Can you work these out from the model? Positions are in its coordinate system, mm. Face numbers are marked on the shaded views. A direction names the side the tool comes from. Round coordinates to 2 decimals unless told otherwise and drop trailing zeros. Write each loop counter-clockwise with the first axis right and the second up, starting at its lowest first coordinate (ties: lowest second). Pieces come first, ordered by that corner, then holes.
Q1. If we section it at A-A (y = 0): Please give me the cut outline in (x, z).
Q2. For the marked faces 1, 2, 3, 4 and 5, which set-ups out of +Z, -Z, +X, -X, +Y, -Y let a thin tool reach every point of the face, with its end or its side?
Q3. We'd pull the mould along Y, two halves only. Please class the marked faces 6, 7 and 8: +Y half, -Y half, draft (parallel to the pull), parting line (faces both ways), or undercut.
Q4. I'm going to push flat-ended pins straight in: pin 1 Ø5 at (x, z) = (0.5, 7) entering from -Y; pin 2 Ø7 at (y, z) = (3.5, 10) entering from -X; pin 3 Ø8 at (x, y) = (16.5, 15.5) entering from +Z; pin 4 Ø4 at (y, z) = (1.5, 5) entering from -X. Where does each tip first touch, or does it pass through?
Q5. If we section it at B-B (z = 10.75): Please give me the cut outline in (x, y), plus the area to 3 significant figures.
Q6. If we section it at D-D (z = 3): Please give me the cut outline in (x, y), plus the area to 3 significant figures.
Q7. Please list where these lines run through material, in increasing order: line 1 along X through (y, z) = (-2.5, 10.25); line 2 along Z through (x, y) = (8.5, 15).
from build123d import *

# Parameters (mm, degrees)
BOX001_W        = 10.2
BOX001_H        = 10.2
BOX001_DEPTH    = 12.5
CHAMFER002_SIZE = 2
BOX_W           = 20
BOX_H           = 20
BOX_DEPTH       = 10
CHAMFER_SIZE    = 6
CHAMFER001_SIZE = 2
FILLET001_R     = 1
CYLINDER_R      = 25
CYLINDER_DEPTH  = 5
FILLET_R        = 1
FILLET002_R     = 1


with BuildPart() as chamfered_hole:
    # Box001 → Box001 (new body)
    with BuildSketch(Plane(origin=(-5.1, -5.1, 0), x_dir=(1, 0, 0), z_dir=(0, 0, 1))):
        with Locations((5.1, 5.1)):
            Rectangle(BOX001_W, BOX001_H)
    extrude(amount=BOX001_DEPTH)

    # Chamfer002
    chamfer002_edges = [chamfered_hole.edges().sort_by_distance(p)[0] for p in [
        (-5.1, -5.1, 6.25),
        (-5.1, 5.1, 6.25),
        (5.1, -5.1, 6.25),
        (5.1, 5.1, 6.25),
    ]]
    chamfer(chamfer002_edges, length=CHAMFER002_SIZE)


with BuildPart() as fillet001:
    # Box → Box (new body)
    with BuildSketch(Plane(origin=(-10, -10, 5), x_dir=(1, 0, 0), z_dir=(0, 0, 1))):
        with Locations((10, 10)):
            Rectangle(BOX_W, BOX_H)
    extrude(amount=BOX_DEPTH)

    # Chamfer
    chamfer_edges = [fillet001.edges().sort_by_distance(p)[0] for p in [
        (-10, -10, 10),
        (10, -10, 10),
    ]]
    chamfer(chamfer_edges, length=CHAMFER_SIZE)

    # Chamfer001
    chamfer001_edges = [fillet001.edges().sort_by_distance(p)[0] for p in [
        (-10, 10, 10),
        (10, 10, 10),
    ]]
    chamfer(chamfer001_edges, length=CHAMFER001_SIZE)

    # Fillet001
    fillet001_edges = [fillet001.edges().sort_by_distance(p)[0] for p in [
        (-10, 2, 15),
        (-9, 9, 15),
        (-7, -7, 15),
        (0, 10, 15),
        (0, -10, 15),
        (9, 9, 15),
        (7, -7, 15),
        (10, 2, 15),
    ]]
    fillet(fillet001_edges, radius=FILLET001_R)


with BuildPart() as print2_side_with_support:
    # Cylinder → Cylinder (new body)
    with BuildSketch(Plane.XY):
        Circle(CYLINDER_R)
    extrude(amount=CYLINDER_DEPTH)

    # Fillet
    fillet_edges = [print2_side_with_support.edges().sort_by_distance(p)[0] for p in [
        (-25, 0, 5),
        (-25, 0, 0),
    ]]
    fillet(fillet_edges, radius=FILLET_R)

    # Fusion: union Fillet001
    add(fillet001.part)

    # Cut: cut Chamfered hole
    add(chamfered_hole.part, mode=Mode.SUBTRACT)

    # Fillet002
    fillet002_edges = [print2_side_with_support.edges().sort_by_distance(p)[0] for p in [
        (0, -5.1, 0),
        (4.1, -4.1, 0),
        (5.1, 0, 0),
        (4.1, 4.1, 0),
        (0, 5.1, 0),
        (-4.1, 4.1, 0),
        (-5.1, 0, 0),
        (-4.1, -4.1, 0),
    ]]
    fillet(fillet002_edges, radius=FILLET002_R)


solid = print2_side_with_support.part
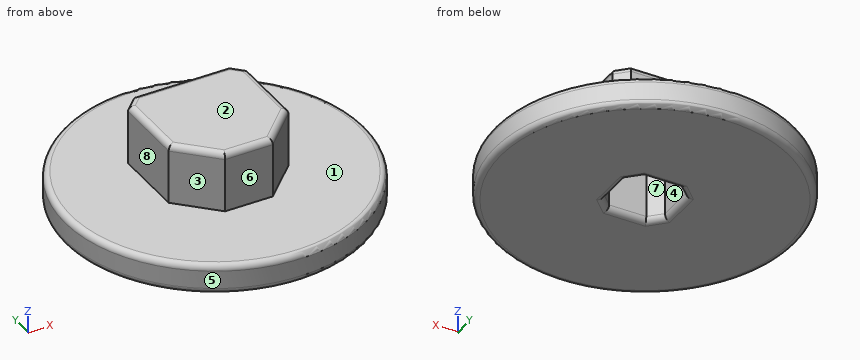
A:
1. outline: (-25, 1) arc R1 ccw to (-24, 0) - (-6.1, 0) arc R1 ccw to (-5.1, 1) - (-5.1, 12.5) - (5.1, 12.5) - (5.1, 1) arc R1 ccw to (6.1, 0) - (24, 0) arc R1 ccw to (25, 1) - (25, 4) arc R1 ccw to (24, 5) - (10, 5) - (10, 14) arc R1 ccw to (9, 15) - (-9, 15) arc R1 ccw to (-10, 14) - (-10, 5) - (-24, 5) arc R1 ccw to (-25, 4) - close
2. face 1: +Z
2. face 2: +Z, +X, -X, +Y, -Y
2. face 3: +Z, -X, -Y
2. face 4: -Z
2. face 5: +Z, -Z
3. face 6: -Y half
3. face 7: undercut
3. face 8: draft
4. pin 1: stops at y = -24.86
4. pin 2: stops at x = -10
4. pin 3: stops at z = 5
4. pin 4: stops at x = -25
5. outline: (-10, -4) - (-4, -10) - (4, -10) - (10, -4) - (10, 8) - (8, 10) - (-8, 10) - (-10, 8) - close; hole (-5.1, -3.1) - (-3.1, -5.1) - (3.1, -5.1) - (5.1, -3.1) - (5.1, 3.1) - (3.1, 5.1) - (-3.1, 5.1) - (-5.1, 3.1) - close
5. area: 264 mm2
6. outline: circle Ø50 at (0, 0); hole (-5.1, -3.1) - (-3.1, -5.1) - (3.1, -5.1) - (5.1, -3.1) - (5.1, 3.1) - (3.1, 5.1) - (-3.1, 5.1) - (-5.1, 3.1) - close
6. area: 1,870 mm2
7. line 1: x = -10 to -5.1, 5.1 to 10
7. line 2: z = 0 to 5
